from build123d import *

# Parameters (mm, degrees)
SKETCH1_W           = 120
SKETCH1_H           = 465
BOSS_EXTRUDE1_DEPTH = 6
SKETCH2_W           = 30
SKETCH2_H           = 20
CUT_EXTRUDE1_DEPTH  = 8
SKETCH4_W           = 20
SKETCH4_H           = 10
SKETCH4_W_2         = 4
SKETCH4_H_2         = 50
BOSS_EXTRUDE2_DEPTH = 6
SKETCH5_W           = 18
SKETCH5_H           = 20
CUT_EXTRUDE2_DEPTH  = 10


with BuildPart() as part:
    # Sketch1 → Boss-Extrude1 (new body)
    with BuildSketch(Plane.XY):
        Rectangle(SKETCH1_W, SKETCH1_H)
    extrude(amount=BOSS_EXTRUDE1_DEPTH)

    # Sketch2 → Cut-Extrude1 (cut)
    with BuildSketch(Plane.XY.offset(6)):
        Polygon((-12, 190), (-42, 190), (-42, 180), (-42, 170), (-12, 170), align=None)
        Polygon((-12, 145), (-42, 145), (-42, 135), (-42, 125), (-12, 125), align=None)
        with Locations((-27, 90)):
            Rectangle(SKETCH2_W, SKETCH2_H)
        with Locations((-27, 45)):
            Rectangle(SKETCH2_W, SKETCH2_H)
        with Locations((-27, 0)):
            Rectangle(SKETCH2_W, SKETCH2_H)
        with Locations((-27, -45)):
            Rectangle(SKETCH2_W, SKETCH2_H)
        with Locations((-27, -90)):
            Rectangle(SKETCH2_W, SKETCH2_H)
        with Locations((-27, -135)):
            Rectangle(SKETCH2_W, SKETCH2_H)
        with Locations((-27, -180)):
            Rectangle(SKETCH2_W, SKETCH2_H)
    extrude(amount=-CUT_EXTRUDE1_DEPTH, mode=Mode.SUBTRACT)

    # Sketch4 → Boss-Extrude2 (add)
    with BuildSketch(Plane.XY.offset(6)):
        with Locations((-30, 232.5)):
            Rectangle(SKETCH4_W, SKETCH4_H)
        with Locations((0, 232.5)):
            Rectangle(SKETCH4_W, SKETCH4_H)
        with Locations((30, 232.5)):
            Rectangle(SKETCH4_W, SKETCH4_H)
        with Locations((-30, -232.5)):
            Rectangle(SKETCH4_W, SKETCH4_H)
        with Locations((0, -232.5)):
            Rectangle(SKETCH4_W, SKETCH4_H)
        with Locations((30, -232.5)):
            Rectangle(SKETCH4_W, SKETCH4_H)
        with Locations((60, 139.5)):
            Rectangle(SKETCH4_W_2, SKETCH4_H_2)
        with Locations((60, 46.5)):
            Rectangle(SKETCH4_W_2, SKETCH4_H_2)
        with Locations((60, -46.5)):
            Rectangle(SKETCH4_W_2, SKETCH4_H_2)
        with Locations((60, -139.5)):
            Rectangle(SKETCH4_W_2, SKETCH4_H_2)
    extrude(amount=-BOSS_EXTRUDE2_DEPTH)

    # Sketch5 → Cut-Extrude2 (cut)
    with BuildSketch(Plane.XY.offset(6)):
        with Locations((-51, 180)):
            Rectangle(SKETCH5_W, SKETCH5_H)
        with Locations((-51, 135)):
            Rectangle(SKETCH5_W, SKETCH5_H)
        with Locations((-51, 90)):
            Rectangle(SKETCH5_W, SKETCH5_H)
        with Locations((-51, 45)):
            Rectangle(SKETCH5_W, SKETCH5_H)
        with Locations((-51, 0)):
            Rectangle(SKETCH5_W, SKETCH5_H)
        with Locations((-51, -45)):
            Rectangle(SKETCH5_W, SKETCH5_H)
        with Locations((-51, -90)):
            Rectangle(SKETCH5_W, SKETCH5_H)
        with Locations((-51, -135)):
            Rectangle(SKETCH5_W, SKETCH5_H)
        with Locations((-51, -180)):
            Rectangle(SKETCH5_W, SKETCH5_H)
    extrude(amount=-CUT_EXTRUDE2_DEPTH, mode=Mode.SUBTRACT)


solid = part.part
Check sheet for the modelled part. Datum: model origin and axes. Units: mm. Round coordinates to 2 decimals unless told otherwise and drop trailing zeros. Loops run counter-clockwise (first coordinate to the right, second up) from the corner with the lowest first, then second, coordinate; pieces in that order, holes last. Notation, with made-up numbers: (84.25, 46) -> (106.25, 46) arc R34 ccw to (106.25, 78) -> close; hole circle Ø10 at (54, 18). An arc over 180 degrees is marked (long way). Put each result on its own line as item: value. Start each with the question number.
1. Section check A-A (x = -47.5). Give the number of separate pieces and of enclosed holes in the cut face, plus the area to 3 significant figures.
2. Gauge pin test, flat ends, axial feed: pin 1 (1.6 mm diameter, centred on x = 61, z = 3, fed in from -Y); pin 2 (1.5 mm diameter, centred on y = -234.5, z = 1.5, fed in from +X); pin 3 (2 mm diameter, centred on x = 12.5, z = 3.5, fed in from +Y). Record the tip position at first contact, or that the pin passes through.
3. Section check B-B (y = 108.5). Enter the section's corners in (x, z).
4. Scan lines: probe 1 along X at (y, z) = (180.5, 3.85); probe 2 along X at (y, z) = (78.5, 2.2); probe 3 along Y at (x, z) = (49, 4.8). Record each from-to range of solid material in increasing order.
5. Section check C-C (x = 14). Enter the section's corners in (y, z).
Findings:
1. separate pieces: 10
1. enclosed holes: 0
1. area: 1,710 mm^2
2. pin 1: stops at y = -164.5
2. pin 2: stops at x = 40
2. pin 3: stops at y = 232.5
3. outline: (-60, 0) -> (60, 0) -> (60, 6) -> (-60, 6) -> close
4. probe 1: x = -12 to 60
4. probe 2: x = -60 to 60
4. probe 3: y = -232.5 to 232.5
5. outline: (-232.5, 0) -> (232.5, 0) -> (232.5, 6) -> (-232.5, 6) -> close
